The listing builds one solid part. Answer for the finished solid, in the listing's coordinates (mm). A direction names the side the tool comes from. Give positions to 0.01 mm unless a question says otherwise; leave off trailing zeros. Write each loop counter-clockwise with the first axis right and the second up, starting at its lowest first coordinate (ties: lowest second). Pieces come first, ordered by that corner, then holes. Notation, with made-up numbers: (64.25, 44.5) - (108.25, 44.5) arc R29 ccw to (108.25, 65.5) - close; hole circle Ø9 at (-15.5, -37). An arc over 180 degrees is marked (long way). One line per question, with ' | ' between items. Start each with the question number.
1. For faces 1 (the face through (17, -0.948, 4)), 2 (the face through (16, 0.552, 4)), determine the directions among +Z, -Z, +X, -X, +Y, -Y from which every point of the face is accessible in a straight line to the end or side of a thin tool.
2. The mould has two halves that part along Y. Classify faces 3 (the face through (-6.53, 1.86, 4.06)), 4 (the face through (-10.54, 6.2, 4.06)), 5 (the face through (16, 0, 0)): +Y half, -Y half, draft (parallel to the pull), parting line (faces both ways), or undercut.
3. A cutting plane is placed at B-B (z = 0.5). State how many separate pieces and enclosed holes the cut face has, then the cut area to 3 significant figures.
4. A cutting plane is placed at A-A (x = 12). Determine the outline of the cut face in (y, z), then the cut area to 3 significant figures.
5. Find the intervals of material crossed by L1, parallel to X at y = 2.5, z = 6.25; L2, parallel to X at y = 3.5, z = 5.25; L3, parallel to Y at x = 20.5, z = 3, in increasing order. Write a range as from..to.
6. Given P1, Ø2, axis at x = 7.5, z = 6.5, coming from the +Y side, flat-ended and moving along its own axis, determine where the tip first touches the part or whether it passes through.
Autodesk Inventor part; units mm, degrees
ref_plane "YZ Plane" through (0, 0, 0) normal (1, 0, 0) x (0, 1, 0)
ref_plane "XZ Plane" through (0, 0, 0) normal (0, 1, 0) x (-1, 0, 0)
ref_plane "XY Plane" through (0, 0, 0) normal (0, 0, 1) x (1, 0, 0)
sketch "Sketch1" plane through (0, 0, 0) normal (0, 0, 1) x (1, 0, 0)
  line L0 (-3.4439, 0.5518) -> (36.5561, 0.5518)
  line L1 (44.5561, -0.9482) -> (-11.4439, -0.9482)
  line L2 (-3.4439, 0.5518) -> (-3.4439, 7.0518)
  line L3 (-3.4439, 7.0518) -> (-11.4439, 7.0518)
  line L4 (36.5561, 0.5518) -> (36.5561, 7.0518)
  line L5 (36.5561, 7.0518) -> (44.5561, 7.0518)
  line L6 (-11.4439, 7.0518) -> (-11.4439, -0.9482)
  line L7 (44.5561, 7.0518) -> (44.5561, -0.9482)
  point P0 (0, 0)
  point P1 (-7.4439, 3.0518)
  point P2 (40.5561, 3.0518)
  dimension "d2" = 8
  dimension "d4" = 8
  dimension "d5" = 1.5
  dimension "d6" = 56
  dimension "d7" = 8
  dimension "d8" = 8
  dimension "d9" = 4
  dimension "d10" = 4
  dimension "d11" = 4
  dimension "d12" = 4
extrude "Extrusion1" add sketch "Sketch1" along normal blind 8
hole "Hole1" at (40.5561, 3.0518, 0) at (-7.4439, 3.0518, 0) direction (0, 0, 1) diameter 3 end through all
fillet "Fillet1" radius 4 2 edges at (-3.4439, 0.5518, 4) (36.5561, 0.5518, 4)
fillet "Fillet2" radius 3 4 edges at (-3.4439, 7.0518, 4) (-11.4439, 7.0518, 4) (44.5561, 7.0518, 4) (36.5561, 7.0518, 4)
fillet "Fillet3" radius 2 2 edges at (44.5561, -0.9482, 4) (-11.4439, -0.9482, 4)
equation "\"d4\" = d2"
equation "\"d7\" = d2"
equation "\"d8\" = d2"
properties part number "3DP_ABS_Bowl_Spring" material "ABS Plastic"
Determined:
1) face 1: +Z, -Z, +X, -X, -Y | face 2: +Z, -Z, +Y
2) face 3: undercut | face 4: +Y half | face 5: draft
3) separate pieces: 1 | enclosed holes: 2 | area: 171 mm2
4) outline: (-0.95, 0) - (0.55, 0) - (0.55, 8) - (-0.95, 8) - close | area: 12.0 mm2
5) L1: -11.44..-8.84, -6.05..-2.88, 35.99..39.16, 41.95..44.56 | L2: -11.44..-8.88, -6.01..-3.3, 36.42..39.12, 41.99..44.56 | L3: -0.95..0.55
6) P1: y = 0.55
